The drawing under review shows one solid part. Ordinate dimensions are in mm from its lowest x, y, z. Give positions to 0.01 mm unless a question says otherwise; leave off trailing zeros. Order: outer loops, then holes, each group sorted by start corner. A loop starts at its lowest first (then second) coordinate and runs counter-clockwise, first axis right, second up. Notation, with made-up numbers: M 77,73 L 103,73 A24 ccw 103,93 Z; hole C 11.5,-24.5 d5. An arc over 180 degrees is marked long. Put each result on its own line as item: value. Start each with the question number.
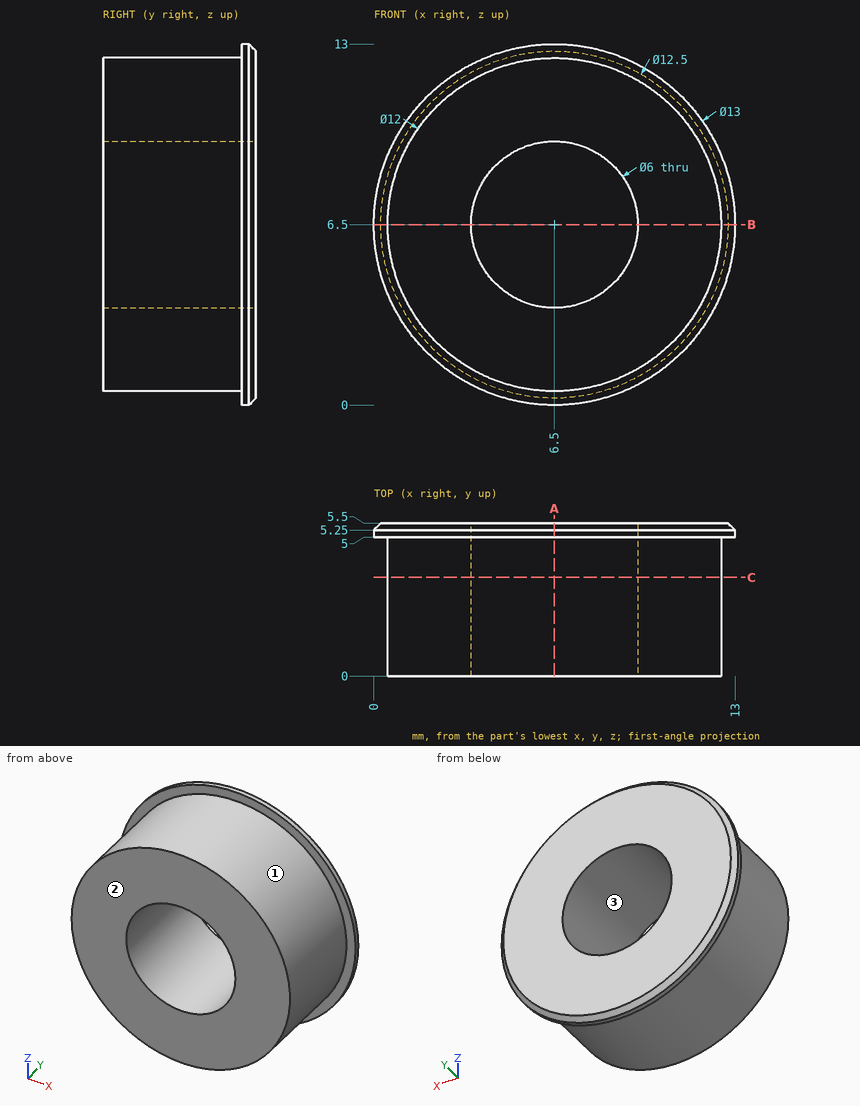
1. Insertion check: pin 1 (1.5 mm diameter, centred on x = 7.5, y = 1, fed in from -Z); pin 2 (1.5 mm diameter, centred on y = 2.5, z = 7, fed in from -X); pin 3 (2 mm diameter, centred on y = 3, z = 2, fed in from +X). Each pin has a flat end and moves straight along its axis. Give the tip position at first contact, or say it passes through.
2. Consider section B-B on z = 6.5. Give the boundary of the cut face in (x, y), then the cut area to 3 significant figures.
3. Consider section C-C on y = 3.55. Give the boundary of the cut face in (x, z).
4. Consider section A-A on x = 6.5. Give the boundary of the cut face in (y, z), then the cut area to 3 significant figures.
5. The part is to be moulded in two halves that separate along Z. For the marked faces 1, 2 and 3, say which applies: +Z half, -Z half, draft (parallel to the pull), parting line (faces both ways), or undercut.
6. To check wall thickness, follow probe 1 along Z at (x, y) = (6.5, 3); probe 2 along Z at (x, y) = (8.25, 3); probe 3 along X at (y, z) = (2.8, 5.25). State the ranges of each line that lie inside material, in increasing order.
Returned:
1. pin 1: stops at z = 0.51
1. pin 2: stops at x = 0.5
1. pin 3: stops at x = 11.37
2. outline: M 0,5 L 0.5,5 L 0.5,0 L 3.5,0 L 3.5,5.5 L 0.25,5.5 L 0,5.25 Z; M 9.5,0 L 12.5,0 L 12.5,5 L 13,5 L 13,5.25 L 12.75,5.5 L 9.5,5.5 Z
2. area: 33.4 mm2
3. outline: C 6.5,6.5 d12; hole C 6.5,6.5 d6
4. outline: M 0,0.5 L 5,0.5 L 5,0 L 5.25,0 L 5.5,0.25 L 5.5,3.5 L 0,3.5 Z; M 0,9.5 L 5.5,9.5 L 5.5,12.75 L 5.25,13 L 5,13 L 5,12.5 L 0,12.5 Z
4. area: 33.4 mm2
5. face 1: parting line
5. face 2: draft
5. face 3: undercut
6. probe 1: z = 0.5 to 3.5, 9.5 to 12.5
6. probe 2: z = 0.76 to 4.06, 8.94 to 12.24
6. probe 3: x = 0.63 to 3.77, 9.23 to 12.37
